The model under review builds one solid part; all positions refer to its coordinate system, in mm. A direction names the side the tool comes from. Coordinates: 2 decimals unless noted, no trailing zeros. Write each loop counter-clockwise with the first axis right and the second up, starting at its lowest first coordinate (ties: lowest second). Pieces come first, ordered by that corner, then holes. Notation, with made-up numbers: (14, 42) - (66, 42) arc R31 cw to (66, 68) - close; hole circle Ø10 at (-6, 43.5). An arc over 180 degrees is marked (long way). Put each result on its own line as item: value. Start each with the question number.
Item 1: Consider section B-B on x = 0. Give the boundary of the cut face in (y, z).
Item 2: Mouldability with a two-part tool opening along Y and no side actions: class faces 1 (the face through (-0.6, 16.29, 3.94)), 2 (the face through (0, -5, 8)), 3 (the face through (-23.977, 1.055, 3.944)) as pulls with the +Y half, pulls with the -Y half, needs draft (parallel to the pull), parting line crosses it, or undercut.
Item 3: Consider section A-A on y = 0. Give the boundary of the cut face in (x, z), then the cut area to 3 significant figures.
Item 4: Consider section C-C on x = 14.5. Give the boundary of the cut face in (y, z).
Item 5: For pin 1 (4 mm diameter, centred on x = 2, z = 5, fed in from -Y); pin 2 (4 mm diameter, centred on x = -20, y = 0, fed in from -Z); pin 3 (1.5 mm diameter, centred on y = 16, z = 2, fed in from -X), all flat-tipped, find the tip position at first contact; note any pin that passes through.
Item 6: Machinability: for faces 4 (the face through (-5.995, -10.384, 3.944)), 5 (the face through (0, -5, 0)), which of the approach directions +Z, -Z, +X, -X, +Y, -Y give a long, thin tool a straight path to every point of the face, cutting with its end or side? Answer none if there is none.
Item 7: To check wall thickness, follow L1, parallel to Y at x = 0, z = 3.5; L2, parallel to X at y = -14, z = 7.75; L3, parallel to Y at x = 14.5, z = 5. State the ranges of each line that lie inside material, in increasing order. Write a range as [from, to].
Item 8: Consider section D-D on z = 6. State how many separate pieces and enclosed holes the cut face has, then the cut area to 3 significant figures.
```python
from build123d import *

# Parameters (mm, degrees)
SKETCH6_R           = 24
BOSS_EXTRUDE1_DEPTH = 8
CUT_EXTRUDE4_DEPTH  = 8
SKETCH7_R           = 4.5
CUT_EXTRUDE5_DEPTH  = 8
SKETCH8_R           = 1.55
CUT_EXTRUDE6_DEPTH  = 8


with BuildPart() as part:
    # Sketch6 → Boss-Extrude1 (new body)
    with BuildSketch(Plane.XY):
        Circle(SKETCH6_R)
    extrude(amount=BOSS_EXTRUDE1_DEPTH)

    # Sketch4 → Cut-Extrude4 (cut)
    with BuildSketch(Plane.XY):
        with BuildLine():
            Line((-3.9, -6.75499815), (-8.15, -14.116214082))
            ThreePointArc((-8.15, -14.116214082), (0, 16.3), (8.15, -14.116214082))
            Line((8.15, -14.116214082), (3.9, -6.75499815))
            ThreePointArc((3.9, -6.75499815), (0, 7.8), (-3.9, -6.75499815))
        make_face()
    extrude(amount=CUT_EXTRUDE4_DEPTH, mode=Mode.SUBTRACT)

    # Sketch7 → Cut-Extrude5 (cut)
    with BuildSketch(Plane(origin=(0, 0, 0), x_dir=(-1, 0, 0), z_dir=(0, 0, -1))):
        Circle(SKETCH7_R)
    extrude(amount=-CUT_EXTRUDE5_DEPTH, mode=Mode.SUBTRACT)

    # Sketch8 → Cut-Extrude6 (cut)
    with BuildSketch(Plane(origin=(0, 0, 0), x_dir=(-1, 0, 0), z_dir=(0, 0, -1))):
        with Locations((0, 20)):
            Circle(SKETCH8_R)
        with Locations((14.142135624, 14.142135624)):
            Circle(SKETCH8_R)
        with Locations((20, 0)):
            Circle(SKETCH8_R)
        with Locations((14.142135624, -14.142135624)):
            Circle(SKETCH8_R)
        with Locations((0, -20)):
            Circle(SKETCH8_R)
        with Locations((-14.142135624, -14.142135624)):
            Circle(SKETCH8_R)
        with Locations((-20, 0)):
            Circle(SKETCH8_R)
        with Locations((-14.142135624, 14.142135624)):
            Circle(SKETCH8_R)
    extrude(amount=-CUT_EXTRUDE6_DEPTH, mode=Mode.SUBTRACT)


solid = part.part
```
Report:
1. outline: (-24, 0) - (-21.55, 0) - (-21.55, 8) - (-24, 8) - close; (-18.45, 0) - (-4.5, 0) - (-4.5, 8) - (-18.45, 8) - close; (4.5, 0) - (7.8, 0) - (7.8, 8) - (4.5, 8) - close; (16.3, 0) - (18.45, 0) - (18.45, 8) - (16.3, 8) - close; (21.55, 0) - (24, 0) - (24, 8) - (21.55, 8) - close
2. face 1: undercut
2. face 2: needs draft
2. face 3: parting line crosses it
3. outline: (-24, 0) - (-21.55, 0) - (-21.55, 8) - (-24, 8) - close; (-18.45, 0) - (-16.3, 0) - (-16.3, 8) - (-18.45, 8) - close; (-7.8, 0) - (-4.5, 0) - (-4.5, 8) - (-7.8, 8) - close; (4.5, 0) - (7.8, 0) - (7.8, 8) - (4.5, 8) - close; (16.3, 0) - (18.45, 0) - (18.45, 8) - (16.3, 8) - close; (21.55, 0) - (24, 0) - (24, 8) - (21.55, 8) - close
3. area: 126 mm²
4. outline: (-19.12, 0) - (-15.65, 0) - (-15.65, 8) - (-19.12, 8) - close; (-12.63, 0) - (-7.45, 0) - (-7.45, 8) - (-12.63, 8) - close; (7.45, 0) - (12.63, 0) - (12.63, 8) - (7.45, 8) - close; (15.65, 0) - (19.12, 0) - (19.12, 8) - (15.65, 8) - close
5. pin 1: y = -24
5. pin 2: z = 0
5. pin 3: x = -18.53
6. face 4: +Z, -Z
6. face 5: -Z, +X, -X, +Y, -Y
7. L1: [-24, -21.55], [-18.45, -4.5], [4.5, 7.8], [16.3, 18.45], [21.55, 24]
7. L2: [-19.49, -15.69], [-12.6, -8.35], [-8.08, 8.08], [8.35, 12.6], [15.69, 19.49]
7. L3: [-19.12, -15.65], [-12.63, -7.45], [7.45, 12.63], [15.65, 19.12]
8. separate pieces: 1
8. enclosed holes: 10
8. area: 1,150 mm²
